Work out the finished part from the listing and answer in its coordinate system (mm). A direction names the side the tool comes from. Coordinates: 2 decimals unless noted, no trailing zeros. Order: outer loops, then holes, each group sorted by start corner. A loop starts at its lowest first (then second) coordinate and runs counter-clockwise, first axis right, second up. Notation, with made-up numbers: M -12,2.25 L 5,2.25 A19 cw 5,29.25 Z; hole C -14,-19.75 d11. An arc over 180 degrees is marked long. Write item = value, one per line. Start each with the question number.
Q1. Each of these flat-tipped pins is pushed along its axis until it touches: P1, Ø17, axis at x = 0, y = 0, coming from the -Z side; P2, Ø3, axis at y = -16, z = 4, coming from the +X side; P3, Ø4, axis at x = 8.5, z = 4.5, coming from the +Y side; P4, Ø6, axis at x = 15.5, z = 10.5, coming from the -Y side. Where does it stop, or does it pass through?
Q2. Straight lines are drawn through the part: line 1 along Y through (x, z) = (0, 9.75) (3 decimals); line 2 along Z through (x, y) = (9, 20); line 3 along X through (y, z) = (-7.5, 2.5). For each, find the intervals that lie inside material, in ascending order.
Q3. Find section B-B on y = 0. Give the vertices of the cut face in (x, z) (3 decimals), and give its area (3 significant figures).
Q4. A tool of negligible diameter and unlimited length cuts with its end or side. For faces 1 (the flat face through (-10, 11, 0)), 2 (the flat face through (-14.1, 14.3, 4)), from which of +Z, -Z, +X, -X, +Y, -Y can it reach the whole face along a straight path? Write none if from no direction.
Q5. Find section A-A on x = 0. Give the vertices of the cut face in (y, z) (3 decimals), and give its area (3 significant figures).
Q6. Find section C-C on z = 2.75. Give the vertices of the cut face in (x, y), and give its area (3 significant figures).
Q7. Find section D-D on x = 16. Give the vertices of the cut face in (y, z), and give its area (3 significant figures).
```python
from build123d import *

# Parameters (mm, degrees)
F0_R     = 19.715
F0_R_2   = 18.38
F1_DEPTH = 4
F0_R_3   = 14.16
F2_DEPTH = 20


with BuildPart() as f1:
    # F0 (on Top) → F1 (new body)
    with BuildSketch(Plane.XY):
        with BuildLine():
            Line((20.97, -11.5905435593), (20.97, 11.5905435593))
            ThreePointArc((20.97, 11.5905435593), (0, 23.96), (-20.97, 11.5905435593))
            Line((-20.97, 11.5905435593), (-20.97, -11.5905435593))
            ThreePointArc((-20.97, -11.5905435593), (0, -23.96), (20.97, -11.5905435593))
        make_face()
        Circle(F0_R, mode=Mode.SUBTRACT)
        Circle(F0_R)
        Circle(F0_R_2, mode=Mode.SUBTRACT)
    extrude(amount=F1_DEPTH)

    # F0 (on Top) → F2 (join)
    with BuildSketch(Plane.XY):
        Circle(F0_R)
        Circle(F0_R_2, mode=Mode.SUBTRACT)
        Circle(F0_R_2)
        Circle(F0_R_3, mode=Mode.SUBTRACT)
    extrude(amount=F2_DEPTH)


solid = f1.part
```
Findings below:
q1.P1 = through
q1.P2 = 19.07
q1.P3 = 23.04
q1.P4 = -15.25
q2.line_1 = -19.715 to -14.16, 14.16 to 19.715
q2.line_2 = 0 to 4
q2.line_3 = -20.97 to -12.01, 12.01 to 20.97
q3.outline = M -20.97,0 L -14.16,0 L -14.16,20 L -19.715,20 L -19.715,4 L -20.97,4 Z; M 14.16,0 L 20.97,0 L 20.97,4 L 19.715,4 L 19.715,20 L 14.16,20 Z
q3.area = 232 mm^2
q4.face_1 = -Z, +X, -X, +Y, -Y
q4.face_2 = +Z
q5.outline = M -23.96,0 L -14.16,0 L -14.16,20 L -19.715,20 L -19.715,4 L -23.96,4 Z; M 14.16,0 L 23.96,0 L 23.96,4 L 19.715,4 L 19.715,20 L 14.16,20 Z
q5.area = 256 mm^2
q6.outline = M -20.97,-11.59 A23.96 ccw 20.97,-11.59 L 20.97,11.59 A23.96 ccw -20.97,11.59 Z; hole C 0,0 d28.32
q6.area = 1,080 mm^2
q7.outline = M -17.83,0 L 17.83,0 L 17.83,4 L 11.52,4 L 11.52,20 L -11.52,20 L -11.52,4 L -17.83,4 Z
q7.area = 511 mm^2
